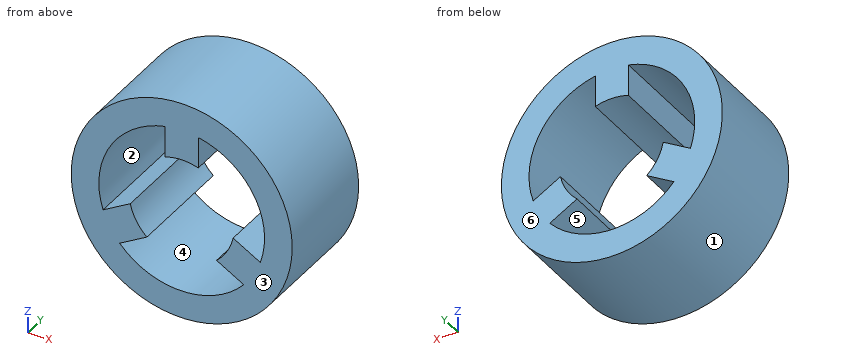
```python
from build123d import *

# Parameters (mm, degrees)
F0_R     = 5.08
F1_DEPTH = 5.08


with BuildPart() as f1:
    # F0 (on Front) → F1 (new body)
    with BuildSketch(Plane.XZ):
        Circle(F0_R)
        with BuildLine():
            ThreePointArc((-0.762, 2.289525), (0, 2.413), (0.762, 2.289525))
            Line((0.762, 2.289525), (0.762, 3.733022))
            ThreePointArc((0.762, 3.733022), (3.299557, 1.905), (3.613892, -1.2066))
            Line((3.613892, -1.2066), (2.363787, -0.484851))
            ThreePointArc((2.363787, -0.484851), (2.089719, -1.2065), (1.601787, -1.804674))
            Line((1.601787, -1.804674), (2.851892, -2.526423))
            ThreePointArc((2.851892, -2.526423), (0, -3.81), (-2.851892, -2.526423))
            Line((-2.851892, -2.526423), (-1.601787, -1.804674))
            ThreePointArc((-1.601787, -1.804674), (-2.089719, -1.2065), (-2.363787, -0.484851))
            Line((-2.363787, -0.484851), (-3.613892, -1.2066))
            ThreePointArc((-3.613892, -1.2066), (-3.299557, 1.905), (-0.762, 3.733022))
            Line((-0.762, 3.733022), (-0.762, 2.289525))
        make_face(mode=Mode.SUBTRACT)
    extrude(amount=F1_DEPTH)


solid = f1.part
```
CAD build for the part. Positions are in the model's coordinates, mm. Face numbers are marked on the shaded views. A direction names the side the tool comes from. Round coordinates to 2 decimals unless told otherwise and drop trailing zeros. Write each loop counter-clockwise with the first axis right and the second up, starting at its lowest first coordinate (ties: lowest second). Pieces come first, ordered by that corner, then holes.
Item 1: Mould opens along X. For the marked faces 1, 2, 3 and 4 say: released by +X, released by -X, zero draft, split by the parting line, or undercut.
Filled in:
face 1: split by the parting line
face 2: undercut
face 3: zero draft
face 4: undercut
Item 2: Tool access for the marked faces 5 and 6: list every direction of +Z, -Z, +X, -X, +Y, -Y with a clear straight run to the whole face (end or side of a thin tool).
Filled in:
face 5: +Y, -Y
face 6: +Z, -Z, +X, -X, +Y
Item 3: Drop flat-ended pins along their axis: pin 1 Ø1.6 at (y, z) = (-3, 3) entering from -X; pin 2 Ø1.5 at (x, z) = (1.5, 3.5) entering from +Y; pin 3 Ø1.5 at (y, z) = (-4, -2) entering from -X; pin 4 Ø3 at (y, z) = (-4.5, -4) entering from +X. Give the stop position or say it passes through.
Filled in:
pin 1: stops at x = -4.58
pin 2: stops at y = 0
pin 3: stops at x = -4.92
pin 4: stops at x = 4.42
Item 4: Band-saw the part on B-B on y = -0.55. Write the cut outline in (x, z), then the cut area to 3 significant figures.
Filled in:
outline: circle Ø10.16 at (0, 0); hole (-3.61, -1.21) - (-2.36, -0.48) arc R2.41 ccw to (-1.6, -1.8) - (-2.85, -2.53) arc R3.81 ccw to (2.85, -2.53) - (1.6, -1.8) arc R2.41 ccw to (2.36, -0.48) - (3.61, -1.21) arc R3.81 ccw to (0.76, 3.73) - (0.76, 2.29) arc R2.41 ccw to (-0.76, 2.29) - (-0.76, 3.73) arc R3.81 ccw to start
area: 41.9 mm2
Item 5: Band-saw the part on C-C on x = 0. Write the cut outline in (y, z), then the cut area to 3 significant figures.
Filled in:
outline: (-5.08, -5.08) - (0, -5.08) - (0, -3.81) - (-5.08, -3.81) - close; (-5.08, 2.41) - (0, 2.41) - (0, 5.08) - (-5.08, 5.08) - close
area: 20.0 mm2
Item 6: Band-saw the part on A-A on z = 0. Write the cut outline in (x, y), then the cut area to 3 significant figures.
Filled in:
outline: (-5.08, -5.08) - (-3.81, -5.08) - (-3.81, 0) - (-5.08, 0) - close; (3.81, -5.08) - (5.08, -5.08) - (5.08, 0) - (3.81, 0) - close
area: 12.9 mm2
Item 7: Drill centre lines: L1, parallel to Z at x = -2.75, y = -3.05; L2, parallel to Z at x = 1.75, y = -3.6; L3, parallel to X at y = -3.1, z = -0.75. Where is each one in solid material? Low to high.
Filled in:
L1: z = -4.27 to -2.64, -2.47 to -0.71, 2.64 to 4.27
L2: z = -4.77 to -3.38, -1.89 to -1.66, 3.38 to 4.77
L3: x = -5.02 to -3.74, -2.82 to -2.29, 2.29 to 2.82, 3.74 to 5.02
Item 8: Band-saw the part on D-D on x = -4. Write the cut outline in (y, z).
Filled in:
outline: (-5.08, -3.13) - (0, -3.13) - (0, 3.13) - (-5.08, 3.13) - close
